```python
from build123d import *

# Parameters (mm, degrees)
ESBO_O2_W                = 84
ESBO_O2_H                = 20
ESBO_O2_R                = 0.75
ESBO_O2_R_2              = 1.4
RESSALTO_EXTRUS_O1_DEPTH = 19
ESBO_O3_W                = 32
ESBO_O3_H                = 51
ESBO_O3_H_2              = 22
CORTE_EXTRUS_O1_DEPTH    = 21
ESBO_O6_W                = 7
ESBO_O6_H                = 5
RESSALTO_EXTRUS_O2_DEPTH = 10
CORTE_EXTRUS_O2_REACH    = 86
ESBO_O4_R                = 0.75
ESBO_O4_R_2              = 1.25
ESBO_O4_R_3              = 2.15
ESBO_O4_R_4              = 1.15


with BuildPart() as part:
    # Esboço2 → Ressalto-extrusão1 (new body, symmetric)
    with BuildSketch(Plane(origin=(0, 0, 0), x_dir=(0, 0, -1), z_dir=(1, 0, 0))):
        with Locations((-2, 0)):
            Rectangle(ESBO_O2_W, ESBO_O2_H)
        with Locations((2.25, 4.25)):
            Circle(ESBO_O2_R, mode=Mode.SUBTRACT)
        with Locations((2.25, -4.25)):
            Circle(ESBO_O2_R, mode=Mode.SUBTRACT)
        with Locations((20, 0)):
            Circle(ESBO_O2_R_2, mode=Mode.SUBTRACT)
    extrude(amount=RESSALTO_EXTRUS_O1_DEPTH, both=True)

    # Esboço3 → Corte-extrusão1 (cut, through all)
    with BuildSketch(Plane(origin=(0, 10, 0), x_dir=(1, 0, 0), z_dir=(0, 1, 0))):
        with Locations((0, 11.5)):
            Rectangle(ESBO_O3_W, ESBO_O3_H)
        with Locations((0, -28)):
            Rectangle(ESBO_O3_W, ESBO_O3_H_2)
    extrude(amount=-CORTE_EXTRUS_O1_DEPTH, mode=Mode.SUBTRACT)

    # Esboço6 → Ressalto-extrusão2 (add)
    with BuildSketch(Plane.XZ.offset(10)):
        with Locations((-15.5, 41.5)):
            Rectangle(ESBO_O6_W, ESBO_O6_H)
        with Locations((15.5, 41.5)):
            Rectangle(ESBO_O6_W, ESBO_O6_H)
    extrude(amount=RESSALTO_EXTRUS_O2_DEPTH)

    # Esboço4 → Corte-extrusão2 (cut, up to next)
    with BuildSketch(Plane.XY.offset(44), mode=Mode.PRIVATE) as corte_extrus_o2_sk1:
        with Locations((0, 3.464101615)):
            Circle(ESBO_O4_R)
    corte_extrus_o2_tool1 = extrude(corte_extrus_o2_sk1.sketch, amount=-CORTE_EXTRUS_O2_REACH, mode=Mode.PRIVATE) & part.part
    add(corte_extrus_o2_tool1.solids().sort_by_distance((0, 3.464102, 44))[0], mode=Mode.SUBTRACT)
    # Esboço4 → Corte-extrusão2 (cut, up to next)
    with BuildSketch(Plane.XY.offset(44), mode=Mode.PRIVATE) as corte_extrus_o2_sk2:
        with Locations((3, -1.732050808)):
            Circle(ESBO_O4_R)
    corte_extrus_o2_tool2 = extrude(corte_extrus_o2_sk2.sketch, amount=-CORTE_EXTRUS_O2_REACH, mode=Mode.PRIVATE) & part.part
    add(corte_extrus_o2_tool2.solids().sort_by_distance((3, -1.732051, 44))[0], mode=Mode.SUBTRACT)
    # Esboço4 → Corte-extrusão2 (cut, up to next)
    with BuildSketch(Plane.XY.offset(44), mode=Mode.PRIVATE) as corte_extrus_o2_sk3:
        with Locations((-3, -1.732050808)):
            Circle(ESBO_O4_R)
    corte_extrus_o2_tool3 = extrude(corte_extrus_o2_sk3.sketch, amount=-CORTE_EXTRUS_O2_REACH, mode=Mode.PRIVATE) & part.part
    add(corte_extrus_o2_tool3.solids().sort_by_distance((-3, -1.732051, 44))[0], mode=Mode.SUBTRACT)
    # Esboço4 → Corte-extrusão2 (cut, up to next)
    with BuildSketch(Plane.XY.offset(44), mode=Mode.PRIVATE) as corte_extrus_o2_sk4:
        with Locations((0, -7.5)):
            Circle(ESBO_O4_R_2)
    corte_extrus_o2_tool4 = extrude(corte_extrus_o2_sk4.sketch, amount=-CORTE_EXTRUS_O2_REACH, mode=Mode.PRIVATE) & part.part
    add(corte_extrus_o2_tool4.solids().sort_by_distance((0, -7.5, 44))[0], mode=Mode.SUBTRACT)
    # Esboço4 → Corte-extrusão2 (cut, up to next)
    with BuildSketch(Plane.XY.offset(44), mode=Mode.PRIVATE) as corte_extrus_o2_sk5:
        Circle(ESBO_O4_R_3)
    corte_extrus_o2_tool5 = extrude(corte_extrus_o2_sk5.sketch, amount=-CORTE_EXTRUS_O2_REACH, mode=Mode.PRIVATE) & part.part
    add(corte_extrus_o2_tool5.solids().sort_by_distance((0, 0, 44))[0], mode=Mode.SUBTRACT)
    # Esboço4 → Corte-extrusão2 (cut, up to next)
    with BuildSketch(Plane.XY.offset(44), mode=Mode.PRIVATE) as corte_extrus_o2_sk6:
        with Locations((-14.5, -15)):
            Circle(ESBO_O4_R_4)
    corte_extrus_o2_tool6 = extrude(corte_extrus_o2_sk6.sketch, amount=-CORTE_EXTRUS_O2_REACH, mode=Mode.PRIVATE) & part.part
    add(corte_extrus_o2_tool6.solids().sort_by_distance((-14.5, -15, 44))[0], mode=Mode.SUBTRACT)
    # Esboço4 → Corte-extrusão2 (cut, up to next)
    with BuildSketch(Plane.XY.offset(44), mode=Mode.PRIVATE) as corte_extrus_o2_sk7:
        with Locations((14.5, -15)):
            Circle(ESBO_O4_R_4)
    corte_extrus_o2_tool7 = extrude(corte_extrus_o2_sk7.sketch, amount=-CORTE_EXTRUS_O2_REACH, mode=Mode.PRIVATE) & part.part
    add(corte_extrus_o2_tool7.solids().sort_by_distance((14.5, -15, 44))[0], mode=Mode.SUBTRACT)


solid = part.part
```
Could you check a few things on this model? Use its own coordinates, in mm. A direction names the side the tool comes from. Round coordinates to 2 decimals unless told otherwise and drop trailing zeros. Loops run counter-clockwise (first coordinate to the right, second up) from the corner with the lowest first, then second, coordinate; pieces in that order, holes last. Notation, with made-up numbers: (-22, -5.5) -> (16, -5.5) arc R27 cw to (16, 26.5) -> close; hole circle Ø6 at (-3.75, -32). An arc over 180 degrees is marked (long way). One line per question, with ' | ' between items.
(1) For faces 1 (the face through (-16, 0, -11)), 2 (the face through (-0.27, -8.72, 41.54)), 3 (the face through (-17.521, -4.915, -2.596)), 4 (the face through (12, -15, 41)), 5 (the face through (-17, -10, -3)), which set-ups out of +Z, -Z, +X, -X, +Y, -Y let a thin tool reach every point of the face, with its end or its side?
Model answer:
face 1: +Y, -Y | face 2: +Z | face 3: +X, -X | face 4: +Z, -Z, -Y | face 5: -Z, +X, -X, -Y
(2) If we section it at A-A on z = 5: List the corners of the cut face in (x, y) for me, and give its area (3 significant figures).
Model answer:
outline: (-19, -10) -> (-16, -10) -> (-16, 10) -> (-19, 10) -> close; (16, -10) -> (19, -10) -> (19, 10) -> (16, 10) -> close | area: 120 mm^2
(3) For pin 1 Ø2.5 at (x, y) = (14.5, -15) entering from -Z; pin 2 Ø3 at (y, z) = (0, -20) entering from +X; pin 3 Ø4 at (x, z) = (10.5, 18) entering from -Y; pin 4 Ø1.4 at (x, y) = (3, -1.73) entering from +Z, each with a flat end and sliding along its axis, tell me the tip position at first contact or that it passes through.
Model answer:
pin 1: stops at z = 39 | pin 2: stops at x = 19 | pin 3: stops at y = -10 | pin 4: stops at z = 17
(4) If I drill on probe 1 along Z at (x, y) = (-11, 3); probe 2 along Y at (x, z) = (0, 41.2); probe 3 along Y at (x, z) = (-17.35, -2.25), over which ranges is the centre line in solid material (lowest first)?
Model answer:
probe 1: z = -40 to -37, 14 to 17, 39 to 44 | probe 2: y = -10 to -8.75, -6.25 to -2.15, 2.15 to 2.71, 4.21 to 10 | probe 3: y = -10 to -5, -3.5 to 3.5, 5 to 10
(5) If we section it at B-B on y = -11: List the corners of the cut face in (x, z) for me, and give its area (3 significant figures).
Model answer:
outline: (-19, 39) -> (-12, 39) -> (-12, 44) -> (-19, 44) -> close; (12, 39) -> (19, 39) -> (19, 44) -> (12, 44) -> close | area: 70.0 mm^2
(6) Thinking about a two-plate mould opening in Y: for faces 6 (the face through (15, -20, 42)), 7 (the face through (-19, 2, 1)), 8 (the face through (-3.595, -2.188, 41.535)), which applies, released by +Y, released by -Y, zero draft, split by the parting line, or undercut?
Model answer:
face 6: released by -Y | face 7: zero draft | face 8: undercut
(7) If we section it at D-D on x = -14.5: List the corners of the cut face in (y, z) for me, and give its area (4 significant figures).
Model answer:
outline: (-20, 39) -> (-16.15, 39) -> (-16.15, 44) -> (-20, 44) -> close; (-13.85, 39) -> (10, 39) -> (10, 44) -> (-13.85, 44) -> close; (-10, -40) -> (10, -40) -> (10, -37) -> (-10, -37) -> close; (-10, 14) -> (10, 14) -> (10, 17) -> (-10, 17) -> close | area: 258.5 mm^2
(8) If we section it at C-C on x = -9.5: List the corners of the cut face in (y, z) for me, and give its area (3 significant figures).
Model answer:
outline: (-10, -40) -> (10, -40) -> (10, -37) -> (-10, -37) -> close; (-10, 14) -> (10, 14) -> (10, 17) -> (-10, 17) -> close; (-10, 39) -> (10, 39) -> (10, 44) -> (-10, 44) -> close | area: 220 mm^2
